Drawing for the job (mm, zero at the part's lowest x, y, z). A direction names the side the tool comes from. Give positions to 0.01 mm unless a question says otherwise; leave off trailing zeros. Order: outer loops, then holes, each group sorted by start corner. A loop starts at its lowest first (then second) coordinate and runs counter-clockwise, first axis right, second up. Notation, with made-up numbers: (76, 21) -> (100, 21) arc R24 ccw to (100, 31) -> close; hole circle Ø11 at (74.25, -10). An arc over 180 degrees is marked (long way). Use a Markdown table: item, result. Add a question column.
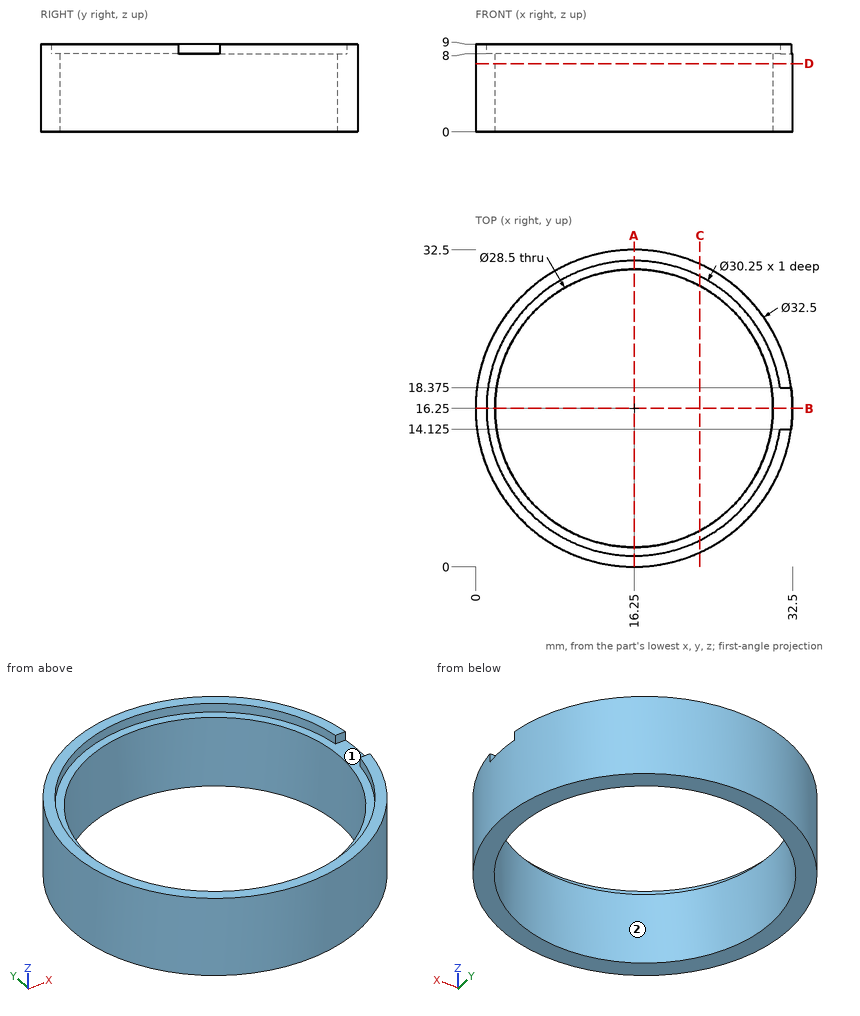
(1) Band-saw the part on B-B on y = 16.25. Give the cut face in (x, z) (3 decimals), plus the area to 3 significant figures.
(2) Tool access for the marked faces 1 and 2: list every direction of +Z, -Z, +X, -X, +Y, -Y with a clear straight run to the whole face (end or side of a thin tool).
(3) Band-saw the part on A-A on x = 16.25. Give the cut face in (y, z) (3 decimals), plus the area to 4 significant figures.
(4) Band-saw the part on D-D on z = 7. Give the cut face in (x, y).
(5) Pin check, flat tips, straight feed: pin 1 Ø1.5 at (x, z) = (18.5, 7.5) entering from +Y; pin 2 Ø1.5 at (x, z) = (5.5, 5.5) entering from -Y; pin 3 Ø5 at (y, z) = (13, 4.5) entering from +X. Stop position of each tip, or through.
(6) Wall check: probe 1 along Y at (x, z) = (16.25, 5); probe 2 along X at (y, z) = (16.25, 8.6) (3 decimals); probe 3 along X at (y, z) = (18, 4.75). Give the ranges that are in metal, low to high.
(7) Band-saw the part on C-C on x = 23. Give the cut face in (y, z), plus the area to 3 significant figures.
Response:
| question | item | result |
|---|---|---|
| 1 | outline | (0, 0) -> (2, 0) -> (2, 8) -> (1.125, 8) -> (1.125, 9) -> (0, 9) -> close; (30.5, 0) -> (32.5, 0) -> (32.5, 8) -> (30.5, 8) -> close |
| 1 | area | 33.1 mm² |
| 2 | face 1 | +Z |
| 2 | face 2 | +Z, -Z |
| 3 | outline | (0, 0) -> (2, 0) -> (2, 8) -> (1.125, 8) -> (1.125, 9) -> (0, 9) -> close; (30.5, 0) -> (32.5, 0) -> (32.5, 9) -> (31.375, 9) -> (31.375, 8) -> (30.5, 8) -> close |
| 3 | area | 34.25 mm² |
| 4 | outline | circle Ø32.5 at (16.25, 16.25); hole circle Ø28.5 at (16.25, 16.25) |
| 5 | pin 1 | stops at y = 32.43 |
| 5 | pin 2 | stops at y = 3.44 |
| 5 | pin 3 | stops at x = 32.48 |
| 6 | probe 1 | y = 0 to 2, 30.5 to 32.5 |
| 6 | probe 2 | x = 0 to 1.125 |
| 6 | probe 3 | x = 0.09 to 2.11, 30.39 to 32.41 |
| 7 | outline | (1.47, 0) -> (3.7, 0) -> (3.7, 8) -> (2.71, 8) -> (2.71, 9) -> (1.47, 9) -> close; (28.8, 0) -> (31.03, 0) -> (31.03, 9) -> (29.79, 9) -> (29.79, 8) -> (28.8, 8) -> close |
| 7 | area | 38.2 mm² |
